Could you check a few things on this model? Use its own coordinates, in mm. A direction names the side the tool comes from. Give positions to 0.01 mm unless a question says otherwise; leave off trailing zeros. Order: outer loops, then holes, each group sorted by start corner. A loop starts at its lowest first (then second) coordinate and runs counter-clockwise, first axis right, second up. Notation, with made-up numbers: (-22.75, 26) - (-7.75, 26) arc R11 ccw to (-7.75, 40) - close; hole circle Ø10 at (-27.75, 42). An arc over 180 degrees is marked (long way). One line per question, with ' | ' between items. Start each with the question number.
1. Imagine slicing it at A-A (z = -31). Please give me the cut outline in (x, y).
2. If we mould it in two halves opening along X, with no side actions, what happens to faces 1 (the cylindrical face through (-3.15, 2.41, -22.21)), 2 (the conical face through (-4.06, -0.9, -2.11)), 3 (the flat face through (-2.072, -1.174, -0.199))? For each: released by +X, released by -X, zero draft, split by the parting line, or undercut.
3. For P1, Ø1.4, axis at x = -0.5, z = 0, coming from the +Y side; P2, Ø3, axis at x = 5.5, y = 2.5, coming from the +Z side; P3, Ø0.8, axis at x = 0.5, z = -1, coming from the -Y side; P4, Ø2, axis at y = -5, z = -22, coming from the +X side, each with a flat end and sliding along its axis, tell me the tip position at first contact or that it passes through.
4. Which directions (+Z, -Z, +X, -X, +Y, -Y) give clear straight access to the entire face, cutting with the end or side of a thin tool? Please do faces 4 (the flat face through (2.072, 1.174, -0.199)), 5 (the flat face through (0, 0, -40.208)), 6 (the cylindrical face through (3.874, -0.86, -2.891)).
5. I need wall thicknesses on probe 1 along Y at (x, z) = (1.5, -2); probe 2 along Y at (x, z) = (-0.25, -38); probe 3 along Z at (x, y) = (0.25, -0.5). Which ranges of each line are inside material? Lowest first, please. Write a range as from..to.
Solid Edge part; units mm, degrees
sketch "Sketch1" plane through (0, 0, 0) normal (1, 0, 0) x (0, 1, 0)
  line L0 (0, -2.1082) -> (0, 2.1082)
  arc A0 (0, 2.1082) -> (6.9469, -2.1082) centre (-0.3606, -6.3169) cw
  line L1 (0, -2.1082) -> (6.9469, -2.1082)
revolve "RevolvedProtrusion1" add sketch "Sketch1" angle 360 about axis through (0, 0, -14.7796) along (0, 0, 1)
sketch "Sketch2" plane through (0, 0, -2.1082) normal (0, 0, -1) x (0, 1, 0)
  circle A0 centre (0, 0) radius 3.9687
extrude "Protrusion1" add sketch "Sketch2" along normal blind 38.1
sketch "Sketch3" plane through (0, 0, -40.2082) normal (0, 0, -1) x (1, 0, 0)
  circle A0 centre (0, 0) radius 3.9662
extrude "Cutout1" cut sketch "Sketch3" against normal blind 36.5125 flip side to cut
sketch "Sketch4" plane through (-0.6032, 0.3606, 4.2164) normal (0, 0, 1) x (1, 0, 0)
  line L0 (-0.7716, 2.0206) -> (1.978, 2.0206)
  line L1 (3.3529, -0.3606) -> (1.978, 2.0206)
  line L2 (1.978, -2.7419) -> (3.3529, -0.3606)
  line L3 (-0.7716, -2.7419) -> (1.978, -2.7419)
  line L4 (-2.1464, -0.3606) -> (-0.7716, -2.7419)
  line L5 (-0.7716, 2.0206) -> (-2.1464, -0.3606)
extrude "ExtrudedCutout_11" cut sketch "Sketch4" against normal blind 6.3246
properties part number "162413"
Results found:
1) outline: circle Ø7.93 at (0, 0)
2) face 1: split by the parting line | face 2: zero draft | face 3: undercut
3) P1: stops at y = 5.91 | P2: stops at z = 0.54 | P3: stops at y = -6.47 | P4: passes through
4) face 4: +Z | face 5: -Z, +X, -X, +Y, -Y | face 6: -Z
5) probe 1: y = -6.72..-2.16, 2.16..6.72 | probe 2: y = -3.96..3.96 | probe 3: z = -40.21..-2.11
